```python
from build123d import *

# Parameters (mm, degrees)
SZKIC1_R                         = 12
DODANIE_WYCI_GNI_CIE3_DEPTH      = 18
DODANIE_WYCI_GNI_CIE3_DEPTH_BACK = 18
SZKIC1_6_W                       = 12
SZKIC1_6_H                       = 90
DODANIE_WYCI_GNI_CIE4_DEPTH      = 45
DODANIE_WYCI_GNI_CIE4_DEPTH_BACK = 45
SKETCH5_R                        = 6.5
CUT_EXTRUDE1_DEPTH               = 12


with BuildPart() as part:
    # Szkic1 → Dodanie-wyci_gni_cie3 (new body, two sides)
    with BuildSketch(Plane.XY) as dodanie_wyci_gni_cie3_sk:
        with BuildLine():
            Line((-788.553538537, 574.11980128), (-837.553538537, 574.11980128))
            Line((-837.553538537, 574.11980128), (-837.553538537, 540.11980128))
            Line((-837.553538537, 540.11980128), (-788.553538537, 540.11980128))
            ThreePointArc((-788.553538537, 540.11980128), (-771.553538537, 557.11980128), (-788.553538537, 574.11980128))
        make_face()
        with Locations((-798.553538537, 557.11980128)):
            Circle(SZKIC1_R, mode=Mode.SUBTRACT)
    extrude(amount=DODANIE_WYCI_GNI_CIE3_DEPTH)
    extrude(dodanie_wyci_gni_cie3_sk.sketch, amount=-DODANIE_WYCI_GNI_CIE3_DEPTH_BACK)

    # Szkic1_6 → Dodanie-wyci_gni_cie4 (add, two sides)
    with BuildSketch(Plane.XY) as dodanie_wyci_gni_cie4_sk:
        with Locations((-843.553538537, 557.11980128)):
            Rectangle(SZKIC1_6_W, SZKIC1_6_H)
    extrude(amount=DODANIE_WYCI_GNI_CIE4_DEPTH)
    extrude(dodanie_wyci_gni_cie4_sk.sketch, amount=-DODANIE_WYCI_GNI_CIE4_DEPTH_BACK)

    # Sketch5 → Cut-Extrude1 (cut)
    with BuildSketch(Plane(origin=(-837.553538537, 0, 0), x_dir=(0, 0, -1), z_dir=(1, 0, 0))):
        with Locations((-35.100505063, 591.220306343)):
            Circle(SKETCH5_R)
        with Locations((35.100505063, 591.220306343)):
            Circle(SKETCH5_R)
        with Locations((35.100505063, 521.019296217)):
            Circle(SKETCH5_R)
        with Locations((-35.100505063, 521.019296217)):
            Circle(SKETCH5_R)
    extrude(amount=-CUT_EXTRUDE1_DEPTH, mode=Mode.SUBTRACT)


solid = part.part
```
Geometry check sheet. Reference: the model listing, model coordinates, mm. A direction names the side the tool comes from. Round coordinates to 2 decimals unless told otherwise and drop trailing zeros. Order: outer loops, then holes, each group sorted by start corner. A loop starts at its lowest first (then second) coordinate and runs counter-clockwise, first axis right, second up. Notation, with made-up numbers: (69, -37.75) -> (84, -37.75) arc R28 cw to (84, -6.75) -> close; hole circle Ø8 at (29, 55). An arc over 180 degrees is marked (long way). Return JSON: item names as keys, results as strings. Group by question number.
Q1. Section check D-D, the plane z = -26. Record the boundary of the cut face in (x, y).
Q2. Section check C-C, the plane z = 16. Record the boundary of the cut face in (x, y), plus the area to 3 significant figures.
Q3. Tool access check on faces 5 (the flat face through (-844, 602.12, 1)), 6 (the flat face through (-812, 557, 18)), 7 (the flat face through (-812, 557, -18)), 8 (the flat face through (-813, 574.12, 0)), 9 (the flat face through (-844, 512.12, 1)). Record the directions out of +Z, -Z, +X, -X, +Y, -Y that give a thin tool (end or side, any length) a straight path to the whole face; none if there is none.
Q4. Section check A-A, the plane y = 519. Record the boundary of the cut face in (x, z).
Q5. Material ranges on probe 1 along X at (y, z) = (523.5, 0); probe 2 along Z at (x, y) = (-833, 556.5); probe 3 along Y at (x, z) = (-790.5, -17.5), recorded low to high. Write a range as from..to.
Q6. Section check B-B, the plane y = 553. Record the boundary of the cut face in (x, z), plus the area to 3 significant figures.
Q7. Gauge pin test, flat ends, axial feed: pin 1 (15 mm diameter, centred on y = 521.02, z = 35.1, fed in from +X); pin 2 (5 mm diameter, centred on x = -780, y = 549, fed in from -Z); pin 3 (5 mm diameter, centred on x = -785.5, z = -7.5, fed in from -Y). Record the tip position at first contact, or that the pin passes through.
Q8. Release check for a two-part mould opening along Y. For faces 1 (the flat face through (-813, 540.12, 0)), 2 (the cylindrical face through (-771.558, 556.746, 0.252)), 3 (the cylindrical face through (-843.47, 527.464, 35.947)), 4 (the cylindrical face through (-808.08, 549.82, -0.25)) record: released by +Y, released by -Y, zero draft, split by the parting line, or undercut.
Numbers:
{
 "1": {"outline": "(-849.55, 512.12) -> (-837.55, 512.12) -> (-837.55, 602.12) -> (-849.55, 602.12) -> close"},
 "2": {"outline": "(-849.55, 512.12) -> (-837.55, 512.12) -> (-837.55, 540.12) -> (-788.55, 540.12) arc R17 ccw to (-788.55, 574.12) -> (-837.55, 574.12) -> (-837.55, 602.12) -> (-849.55, 602.12) -> close; hole circle Ø24 at (-798.55, 557.12)", "area": "2,750 mm^2"},
 "3": {"face 5": "+Z, -Z, +X, -X, +Y", "face 6": "+Z, +X, +Y, -Y", "face 7": "-Z, +X, +Y, -Y", "face 8": "+Z, -Z, +X, +Y", "face 9": "+Z, -Z, +X, -X, -Y"},
 "4": {"outline": "(-849.55, -45) -> (-837.55, -45) -> (-837.55, -41.28) -> (-849.55, -41.28) -> close; (-849.55, -28.92) -> (-837.55, -28.92) -> (-837.55, 28.92) -> (-849.55, 28.92) -> close; (-849.55, 41.28) -> (-837.55, 41.28) -> (-837.55, 45) -> (-849.55, 45) -> close"},
 "5": {"probe 1": "-849.55..-837.55", "probe 2": "-18..18", "probe 3": "540.12..548.22, 566.02..574.12"},
 "6": {"outline": "(-849.55, -45) -> (-837.55, -45) -> (-837.55, -18) -> (-809.82, -18) -> (-809.82, 18) -> (-837.55, 18) -> (-837.55, 45) -> (-849.55, 45) -> close; (-787.28, -18) -> (-772.06, -18) -> (-772.06, 18) -> (-787.28, 18) -> close", "area": "2,630 mm^2"},
 "7": {"pin 1": "x = -837.55", "pin 2": "z = -18", "pin 3": "y = 540.13"},
 "8": {"face 1": "released by -Y", "face 2": "split by the parting line", "face 3": "undercut", "face 4": "undercut"}
}
